Model file for the job. Use its own axes, mm. Round coordinates to 2 decimals unless told otherwise and drop trailing zeros. Loops run counter-clockwise (first coordinate to the right, second up) from the corner with the lowest first, then second, coordinate; pieces in that order, holes last. Notation, with made-up numbers: M 27.5,-10 L 61.5,-10 A16 cw 61.5,12 Z; hole C 15,3 d8. An arc over 180 degrees is marked long. Use a Markdown table: item, result. Add a question column.
Q1. Cut at B-B (x = 69). Give the cut face in (y, z).
Q2. Cut at A-A (y = 70). Give the cut face in (x, z).
Q3. Pin check, flat tips, straight feed: pin 1 (1.5 mm diameter, centred on x = -60, z = 1, fed in from +Y); pin 2 (0.9 mm diameter, centred on y = 68.5, z = 1.5, fed in from -X). Stop position of each tip, or through.
Q4. Cut at C-C (y = 17). State how many separate pieces and enclosed holes the cut face has, plus the area to 3 significant figures.
Q5. Probe line 1 (Y direction, x = -20, z = 1.6); line 2 (X direction, y = 59, z = 0.7); line 3 (X direction, y = 80, z = 2.25). List the from-to ranges inside material, lowest first. Write a range as from..to.
from build123d import *

# Parameters (mm, degrees)
SKETCH_1_R          = 1.55
SKETCH_1_R_2        = 2.65
SKETCH_1_W          = 29
SKETCH_1_H          = 38
SKETCH_1_W_2        = 44
EXTRUDE_1_DEPTH     = 3
SKETCH_4_W          = 20
SKETCH_4_H          = 35
CUT_EXTRUDE_1_DEPTH = 10
SKETCH_3_W          = 18
SKETCH_3_H          = 35
EXTRUDE_2_DEPTH     = 3
SKETCH_5_R          = 1.65
CUT_EXTRUDE_2_DEPTH = 5
CHAMFER_1_SIZE      = 10
FILLET_1_R          = 2
EXTRUDE_1_2_DEPTH   = 3
FILLET_3_R          = 2


with BuildPart() as part:
    # 草图1 → Extrude 1 (new body)
    with BuildSketch(Plane.XY):
        Polygon((-10, 50), (-10, 85), (10, 85), (10, 50), (79, 50), (79, 0), (-79, 0), (-79, 50), align=None)
        with Locations((-6, 81)):
            Circle(SKETCH_1_R, mode=Mode.SUBTRACT)
        with Locations(Location((6, 81, 0), (0, 0, 180))):
            Circle(SKETCH_1_R, mode=Mode.SUBTRACT)
        with Locations((-6, 59)):
            Circle(SKETCH_1_R, mode=Mode.SUBTRACT)
        with Locations(Location((6, 59, 0), (0, 0, 180))):
            Circle(SKETCH_1_R, mode=Mode.SUBTRACT)
        with Locations((-69, 37)):
            Circle(SKETCH_1_R_2, mode=Mode.SUBTRACT)
        with Locations((-69, 7)):
            Circle(SKETCH_1_R_2, mode=Mode.SUBTRACT)
        with Locations(Location((69, 7, 0), (0, 0, 180))):
            Circle(SKETCH_1_R_2, mode=Mode.SUBTRACT)
        with Locations(Location((69, 37, 0), (0, 0, 180))):
            Circle(SKETCH_1_R_2, mode=Mode.SUBTRACT)
        with Locations((-28, 37)):
            Circle(SKETCH_1_R_2, mode=Mode.SUBTRACT)
        with Locations((-28, 7)):
            Circle(SKETCH_1_R_2, mode=Mode.SUBTRACT)
        with Locations(Location((28, 7, 0), (0, 0, 180))):
            Circle(SKETCH_1_R_2, mode=Mode.SUBTRACT)
        with Locations(Location((28, 37, 0), (0, 0, 180))):
            Circle(SKETCH_1_R_2, mode=Mode.SUBTRACT)
        with Locations((-48.5, 25)):
            Rectangle(SKETCH_1_W, SKETCH_1_H, mode=Mode.SUBTRACT)
        with Locations((48.5, 25)):
            Rectangle(SKETCH_1_W, SKETCH_1_H, mode=Mode.SUBTRACT)
        with Locations((0, 25)):
            Rectangle(SKETCH_1_W_2, SKETCH_1_H, mode=Mode.SUBTRACT)
    extrude(amount=EXTRUDE_1_DEPTH)

    # 草图4 → 切除-拉伸1 (cut)
    with BuildSketch(Plane(origin=(0, 0, 0), x_dir=(-1, 0, 0), z_dir=(0, 0, -1))):
        with Locations((0, 67.5)):
            Rectangle(SKETCH_4_W, SKETCH_4_H)
    extrude(amount=-CUT_EXTRUDE_1_DEPTH, mode=Mode.SUBTRACT)

    # 草图3 → 凸台-拉伸2 (add)
    with BuildSketch(Plane(origin=(0, 0, 0), x_dir=(-1, 0, 0), z_dir=(0, 0, -1))):
        with Locations((-20, 67.5)):
            Rectangle(SKETCH_3_W, SKETCH_3_H)
        with Locations((20, 67.5)):
            Rectangle(SKETCH_3_W, SKETCH_3_H)
    extrude(amount=-EXTRUDE_2_DEPTH)

    # 草图5 → 切除-拉伸2 (cut)
    with BuildSketch(Plane(origin=(0, 0, 0), x_dir=(-1, 0, 0), z_dir=(0, 0, -1))):
        with Locations((-20, 80)):
            Circle(SKETCH_5_R)
        with Locations((-20, 70)):
            Circle(SKETCH_5_R)
        with Locations((-20, 60)):
            Circle(SKETCH_5_R)
        with Locations(Location((20, 60, 0), (0, 0, 180))):
            Circle(SKETCH_5_R)
        with Locations(Location((20, 70, 0), (0, 0, 180))):
            Circle(SKETCH_5_R)
        with Locations(Location((20, 80, 0), (0, 0, 180))):
            Circle(SKETCH_5_R)
    extrude(amount=-CUT_EXTRUDE_2_DEPTH, mode=Mode.SUBTRACT)

    # 倒角1
    chamfer_1_edges = [part.edges().sort_by_distance(p)[0] for p in [
        (29, 50, 1.5),
        (-29, 50, 1.5),
    ]]
    chamfer(chamfer_1_edges, length=CHAMFER_1_SIZE)

    # 圆角1
    fillet_1_edges = [part.edges().sort_by_distance(p)[0] for p in [
        (79, 50, 1.5),
        (79, 0, 1.5),
        (-79, 0, 1.5),
        (-79, 50, 1.5),
        (11, 85, 1.5),
        (11, 50, 1.5),
        (29, 85, 1.5),
        (-29, 85, 1.5),
        (-11, 50, 1.5),
        (-11, 85, 1.5),
        (-39, 50, 1.5),
        (-29, 60, 1.5),
        (29, 60, 1.5),
        (39, 50, 1.5),
    ]]
    fillet(fillet_1_edges, radius=FILLET_1_R)

    # 草图6 → Extrude 1 2 (add)
    with BuildSketch(Plane(origin=(0, 0, 0), x_dir=(-1, 0, 0), z_dir=(0, 0, -1))):
        Polygon((-64.192426869, 43.089990021), (-35.192426869, 5.089990021), (-32.807573131, 6.910009979), (-61.807573131, 44.910009979), align=None)
        Polygon((-35.192426869, 44.910009979), (-64.192426869, 6.910009979), (-61.807573131, 5.089990021), (-32.807573131, 43.089990021), align=None)
        Polygon((-22.980429806, 42.864765488), (21.019570194, 4.864765488), (22.980429806, 7.135234512), (-21.019570194, 45.135234512), align=None)
        Polygon((21.019570194, 45.135234512), (-22.980429806, 7.135234512), (-21.019570194, 4.864765488), (22.980429806, 42.864765488), align=None)
        Polygon((32.807573131, 43.089990021), (61.807573131, 5.089990021), (64.192426869, 6.910009979), (35.192426869, 44.910009979), align=None)
        Polygon((61.807573131, 44.910009979), (32.807573131, 6.910009979), (35.192426869, 5.089990021), (64.192426869, 43.089990021), align=None)
    extrude(amount=-EXTRUDE_1_2_DEPTH)

    # 圆角3
    fillet_3_edges = [part.edges().sort_by_distance(p)[0] for p in [
        (35.886908169, 44, 1.5),
        (61.113091831, 44, 1.5),
        (63, 8.472500359, 1.5),
        (63, 41.527499641, 1.5),
        (61.113091831, 6, 1.5),
        (35.886908169, 6, 1.5),
        (34, 41.527499641, 1.5),
        (34, 8.472500359, 1.5),
        (48.5, 22.527499641, 1.5),
        (48.5, 27.472500359, 1.5),
        (46.613091831, 25, 1.5),
        (50.386908169, 25, 1.5),
        (-19.705088128, 44, 1.5),
        (19.705088128, 44, 1.5),
        (22, 7.981969344, 1.5),
        (22, 42.018030656, 1.5),
        (19.705088128, 6, 1.5),
        (-19.705088128, 6, 1.5),
        (-22, 42.018030656, 1.5),
        (-22, 7.981969344, 1.5),
        (0, 23.018030656, 1.5),
        (0, 26.981969344, 1.5),
        (-2.294911872, 25, 1.5),
        (2.294911872, 25, 1.5),
        (-63, 41.527499641, 1.5),
        (-63, 8.472500359, 1.5),
        (-61.113091831, 44, 1.5),
        (-35.886908169, 44, 1.5),
        (-34, 8.472500359, 1.5),
        (-34, 41.527499641, 1.5),
        (-35.886908169, 6, 1.5),
        (-61.113091831, 6, 1.5),
        (-48.5, 22.527499641, 1.5),
        (-48.5, 27.472500359, 1.5),
        (-50.386908169, 25, 1.5),
        (-46.613091831, 25, 1.5),
    ]]
    fillet(fillet_3_edges, radius=FILLET_3_R)


solid = part.part
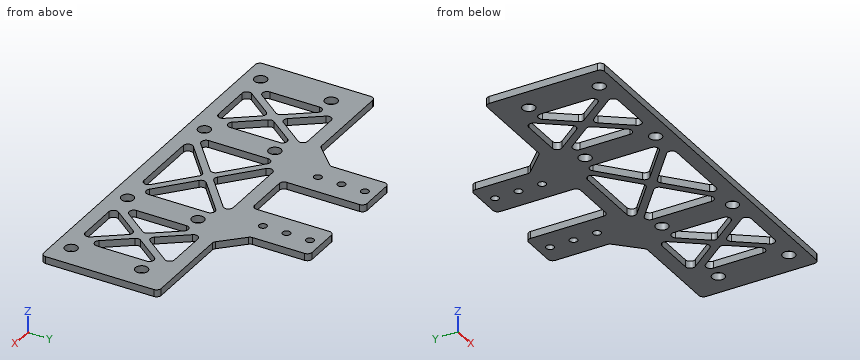
Checked values:
| question | item | result |
|---|---|---|
| 1 | outline | M 0,0 L 4.35,0 L 4.35,3 L 0,3 Z; M 9.65,0 L 34.35,0 L 34.35,3 L 9.65,3 Z; M 39.65,0 L 50,0 L 50,3 L 39.65,3 Z |
| 2 | outline | M -29,0 L -21.65,0 L -21.65,3 L -29,3 Z; M -18.35,0 L -11,0 L -11,3 L -18.35,3 Z; M 11,0 L 18.35,0 L 18.35,3 L 11,3 Z; M 21.65,0 L 29,0 L 29,3 L 21.65,3 Z |
| 3 | pin 1 | stops at y = 50 |
| 3 | pin 2 | stops at x = -29 |
| 4 | separate pieces | 10 |
| 4 | enclosed holes | 0 |
| 4 | area | 241 mm^2 |
| 5 | line 1 | y = 0..10.35, 39.65..58.35, 61.65..68.35, 71.65..78.35, 81.65..85 |
| 5 | line 2 | x = -30..-21.31, -18.69..-11, 11..18.69, 21.31..30 |
| 5 | line 3 | x = -29..-21.65, -18.35..-11, 11..18.35, 21.65..29 |
